Can you work these out from the model? Positions are in its coordinate system, mm. A direction names the side the tool comes from. Give positions to 0.01 mm unless a question says otherwise; leave off trailing zeros. Loops run counter-clockwise (first coordinate to the right, second up) from the corner with the lowest first, then second, coordinate; pieces in that order, holes last. Notation, with made-up numbers: M 32,69.25 L 82,69.25 A23 cw 82,95.25 Z; hole C 61.5,7 d10. An arc over 180 degrees is marked long. Put each result on its own line as item: value. Start each with the question number.
1) Imagine slicing it at C-C (z = 17.5). Write out the boundary of the cut face in (x, y).
2) Imagine slicing it at A-A (y = -22). Write out the boundary of the cut face in (x, z), then the cut area to 3 significant figures.
3) Please list where these lines run through material, in increasing order: line 1 along Z through (x, y) = (-34.5, -15.5); line 2 along X through (y, z) = (-16, 15); line 3 along Y through (x, z) = (-33, 23). Write a range as from..to.
4) For P1, Ø12, axis at x = -15, z = 10.5, coming from the +Y side; P2, Ø5, axis at y = -19.5, z = 21, coming from the -X side; P3, Ø10, axis at y = -21.5, z = 22.5, coming from the +X side; P4, Ø9.5, axis at x = -37.5, z = 22, coming from the -Y side, each with a flat end and sliding along its axis, tell me the tip position at first contact or that it passes through.
5) Imagine slicing it at D-D (x = -11.5). Write out the boundary of the cut face in (y, z), then the cut area to 3 significant figures.
6) For faces 1 (the flat face through (-35, -22, 12.7)), 2 (the flat face through (-3.22, -6.44, 22.36)), 3 (the flat face through (-6, -22, 12.7)), which set-ups out of +Z, -Z, +X, -X, +Y, -Y let a thin tool reach every point of the face, with its end or its side?
7) Imagine slicing it at B-B (x = -2.5). Write out the boundary of the cut face in (y, z), then the cut area to 3 significant figures.
from build123d import *

# Parameters (mm, degrees)
F0_W     = 44.45
F0_H     = 12.7
F1_DEPTH = 31.75
F2_W     = 44.45
F2_H     = 12.7
F3_DEPTH = 19.05
F4_W     = 12.7
F4_H     = 19.05
F5_DEPTH = 19.05
F7_DEPTH = 25.4
F9_DEPTH = 25.4


with BuildPart() as f1:
    # F0 (on Front) → F1 (new body)
    with BuildSketch(Plane.XZ):
        with Locations((-22.225, 6.35)):
            Rectangle(F0_W, F0_H)
    extrude(amount=F1_DEPTH)

    # F2 (on face) → F3 (join)
    with BuildSketch(Plane.XY.offset(12.7)):
        with Locations((-22.225, -6.35)):
            Rectangle(F2_W, F2_H)
    extrude(amount=F3_DEPTH)

    # F4 (on face) → F5 (join)
    with BuildSketch(Plane.XZ.offset(12.7)):
        with Locations((-19.05, 22.225)):
            Rectangle(F4_W, F4_H)
    extrude(amount=F5_DEPTH)

    # F6 (on face) → F7 (cut)
    with BuildSketch(Plane.YZ.offset(-12.7)):
        Polygon((-31.75, 31.75), (-31.75, 12.7), (-12.7, 31.75), align=None)
    extrude(amount=-F7_DEPTH, mode=Mode.SUBTRACT)

    # F8 (on face) → F9 (cut)
    with BuildSketch(Plane.XZ.offset(12.7)):
        Polygon((0, 31.75), (-6.35, 31.75), (0, 12.7), align=None)
    extrude(amount=-F9_DEPTH, mode=Mode.SUBTRACT)


solid = f1.part
Recorded:
1. outline: M -44.45,-12.7 L -25.4,-12.7 L -25.4,-26.95 L -12.7,-26.95 L -12.7,-12.7 L -1.6,-12.7 L -1.6,0 L -44.45,0 Z
2. outline: M -44.45,0 L 0,0 L 0,12.7 L -12.7,12.7 L -12.7,22.45 L -25.4,22.45 L -25.4,12.7 L -44.45,12.7 Z
2. area: 688 mm²
3. line 1: 0..12.7
3. line 2: -25.4..-12.7
3. line 3: -12.7..0
4. P1: y = 0
4. P2: x = -25.4
4. P3: x = -12.7
4. P4: y = -12.7
5. outline: M -31.75,0 L 0,0 L 0,31.75 L -12.7,31.75 L -12.7,12.7 L -31.75,12.7 Z
5. area: 645 mm²
6. face 1: +Z, -X, -Y
6. face 2: +Z, +X, +Y, -Y
6. face 3: +Z, +X, -Y
7. outline: M -31.75,0 L 0,0 L 0,20.2 L -12.7,20.2 L -12.7,12.7 L -31.75,12.7 Z
7. area: 498 mm²
